```python
from build123d import *

# Parameters (mm, degrees)
SKETCH_W            = 100
SKETCH_H            = 70
PAD_DEPTH           = 10
POCKET_DEPTH        = 5
LINEARPATTERN_COUNT = 6
LINEARPATTERN_PITCH = 16


with BuildPart() as part:
    # Sketch → Pad (new body)
    with BuildSketch(Plane.XY):
        Rectangle(SKETCH_W, SKETCH_H)
    extrude(amount=PAD_DEPTH)

    # Sketch001 (on Face6 of Pad) → Pocket (cut)
    with BuildSketch(Plane.XY.offset(10)):
        with BuildLine():
            ThreePointArc((-36, -7), (-40, -3), (-44, -7))
            Line((-44, -7), (-44, -27))
            ThreePointArc((-44, -27), (-40, -31), (-36, -27))
            Line((-36, -7), (-36, -27))
        make_face()
    pocket = extrude(amount=-POCKET_DEPTH, mode=Mode.SUBTRACT)

    # LinearPattern: Pocket ×6
    with Locations(*[(i * LINEARPATTERN_PITCH, 0, 0) for i in range(1, LINEARPATTERN_COUNT)]):
        add(pocket, mode=Mode.SUBTRACT)


solid = part.part
```
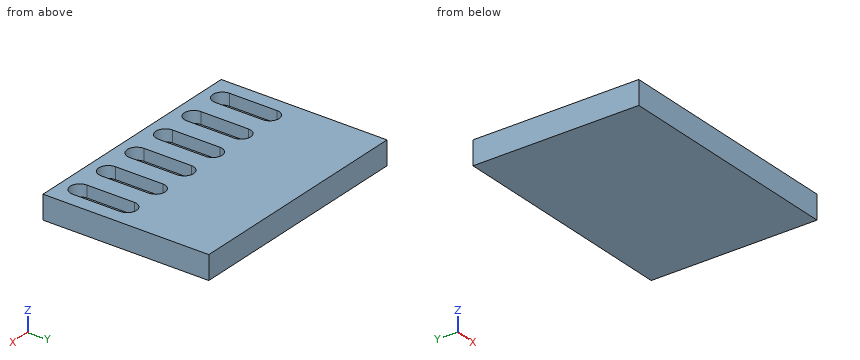
For this review, take the finished solid that the model builds, in its own axes (mm). Coordinates: 2 decimals unless noted, no trailing zeros. Order: outer loops, then holes, each group sorted by start corner. A loop starts at its lowest first (then second) coordinate and runs counter-clockwise, first axis right, second up. Notation, with made-up numbers: (12.5, -7.5) - (56.5, -7.5) arc R30 cw to (56.5, 16.5) - close; hole circle Ø10 at (-27, -10.5). An arc over 180 degrees is marked (long way). Answer as a JSON object with one key per item and string values. Group by question number.
1. We need section D-D on y = -5.5. State the section outline as (x, z) points.
2. We need section C-C on x = -7. State the section outline as (y, z) points, then the cut area to 3 significant figures.
3. We need section B-B on x = 40. State the section outline as (y, z) points, then the cut area to 3 significant figures.
4. For probe 1 along Z at (x, y) = (-37.5, -25), list the stretches that pass through material, from the lowest coordinate up.
5. Clearance check with a flat-ended pin moving along its axis: P1, Ø2.5, axis at x = 40, y = -21.5, coming from the +Z side. State where the tip first meets the part, or that it passes through.
6. We need section A-A on y = -17.5. State the section outline as (x, z) points.
Final values:
{
 "1": {"outline": "(-50, 0) - (50, 0) - (50, 10) - (43.71, 10) - (43.71, 5) - (36.29, 5) - (36.29, 10) - (27.71, 10) - (27.71, 5) - (20.29, 5) - (20.29, 10) - (11.71, 10) - (11.71, 5) - (4.29, 5) - (4.29, 10) - (-4.29, 10) - (-4.29, 5) - (-11.71, 5) - (-11.71, 10) - (-20.29, 10) - (-20.29, 5) - (-27.71, 5) - (-27.71, 10) - (-36.29, 10) - (-36.29, 5) - (-43.71, 5) - (-43.71, 10) - (-50, 10) - close"},
 "2": {"outline": "(-35, 0) - (35, 0) - (35, 10) - (-3.13, 10) - (-3.13, 5) - (-30.87, 5) - (-30.87, 10) - (-35, 10) - close", "area": "561 mm²"},
 "3": {"outline": "(-35, 0) - (35, 0) - (35, 10) - (-3, 10) - (-3, 5) - (-31, 5) - (-31, 10) - (-35, 10) - close", "area": "560 mm²"},
 "4": {"probe 1": "0 to 5"},
 "5": {"P1": "z = 5"},
 "6": {"outline": "(-50, 0) - (50, 0) - (50, 10) - (44, 10) - (44, 5) - (36, 5) - (36, 10) - (28, 10) - (28, 5) - (20, 5) - (20, 10) - (12, 10) - (12, 5) - (4, 5) - (4, 10) - (-4, 10) - (-4, 5) - (-12, 5) - (-12, 10) - (-20, 10) - (-20, 5) - (-28, 5) - (-28, 10) - (-36, 10) - (-36, 5) - (-44, 5) - (-44, 10) - (-50, 10) - close"}
}
